```python
from build123d import *

# Parameters (mm, degrees)
PAD_DEPTH       = 74.5
PAD001_DEPTH    = 1
POCKET_DEPTH    = 28.9
POCKET001_DEPTH = 5.001
SKETCH004_R     = 5
POCKET002_DEPTH = 3
SKETCH005_R     = 2
HOLE_DEPTH      = 25
POCKET003_DEPTH = 117.501


with BuildPart() as part:
    # Sketch → Pad (new body)
    with BuildSketch(Plane.XY):
        with BuildLine():
            Line((1, -1), (1, -5))
            Line((1, -5), (114.5, -5))
            Line((114.5, -1), (114.5, -5))
            ThreePointArc((114.5, -1), (115.914212, -0.414215), (116.5, 0.999995))
            Line((116.5, 0.999995), (116.5, 26.9))
            ThreePointArc((116.5, 26.9), (115.914214, 28.314214), (114.5, 28.9))
            Line((1, 28.9), (114.5, 28.9))
            ThreePointArc((1, 28.9), (-0.414214, 28.314214), (-1, 26.9))
            Line((-1, 1), (-1, 26.9))
            ThreePointArc((-1, 1), (-0.414214, -0.414214), (1, -1))
        make_face()
        with BuildLine():
            Line((1, 0), (114.5, 0))
            ThreePointArc((114.5, 0), (115.207107, 0.292893), (115.5, 1))
            Line((115.5, 1), (115.5, 26.9))
            ThreePointArc((115.5, 26.9), (115.207107, 27.607107), (114.5, 27.9))
            Line((114.5, 27.9), (1, 27.9))
            ThreePointArc((1, 27.9), (0.292893, 27.607107), (0, 26.9))
            Line((0, 26.9), (0, 1))
            ThreePointArc((0, 1), (0.292893, 0.292893), (1, 0))
        make_face(mode=Mode.SUBTRACT)
    extrude(amount=PAD_DEPTH)

    # Sketch001 → Pad001 (join)
    with BuildSketch(Plane.XY):
        with BuildLine():
            Line((-1, 1), (-1, 26.9))
            ThreePointArc((1, 28.9), (-0.414214, 28.314214), (-1, 26.9))
            Line((1, 28.9), (114.5, 28.9))
            ThreePointArc((116.5, 26.9), (115.914214, 28.314214), (114.5, 28.9))
            Line((116.5, 26.9), (116.5, 0.999995))
            ThreePointArc((114.5, -1), (115.914212, -0.414215), (116.5, 0.999995))
            Line((114.5, -1), (114.5, -5))
            Line((114.5, -5), (1, -5))
            Line((1, -5), (1, -1))
            ThreePointArc((-1, 1), (-0.414214, -0.414214), (1, -1))
        make_face()
        Polygon((9, 26.9), (9, 1), (106.5, 0.999995), (106.5, 26.9), align=None, mode=Mode.SUBTRACT)
    extrude(amount=PAD001_DEPTH)

    # Sketch002 (on Face22 of Pad001) → Pocket (cut)
    with BuildSketch(Plane(origin=(0, 28.9, 0), x_dir=(-1, 0, 0), z_dir=(0, 1, 0))):
        Polygon((-104.5, 21), (-104.5, 61), (-124.5, 61), (-124.5, 74.5), (9, 74.5), (9, 61), (-11, 61), (-11, 21), align=None)
    extrude(amount=-POCKET_DEPTH, mode=Mode.SUBTRACT)

    # Sketch003 (on Face30 of Pocket) → Pocket001 (cut, through all)
    with BuildSketch(Plane(origin=(0, 0, 0), x_dir=(-1, 0, 0), z_dir=(0, 1, 0))):
        with BuildLine():
            ThreePointArc((-101, 74.5), (-110.545942, 70.545942), (-114.5, 61))
            Line((-114.5, 61), (-124.5, 61))
            Line((-124.5, 61), (-124.5, 74.5))
            Line((-124.5, 74.5), (-101, 74.5))
        make_face()
        with BuildLine():
            ThreePointArc((-1, 61), (-4.954058, 70.545942), (-14.5, 74.5))
            Line((-14.5, 74.5), (9, 74.5))
            Line((9, 74.5), (9, 61))
            Line((9, 61), (-1, 61))
        make_face()
    extrude(amount=-POCKET001_DEPTH, mode=Mode.SUBTRACT)

    # Sketch004 (on Face42 of Pocket001) → Pocket002 (cut)
    with BuildSketch(Plane(origin=(0, 0, 0), x_dir=(-1, 0, 0), z_dir=(0, 1, 0))):
        with Locations((-84.5, 41)):
            Circle(SKETCH004_R)
        with Locations((-31, 41)):
            Circle(SKETCH004_R)
    extrude(amount=-POCKET002_DEPTH, mode=Mode.SUBTRACT)

    # Sketch005 (on Face42 of Pocket001) → Hole (cut)
    with BuildSketch(Plane(origin=(0, 0, 0), x_dir=(-1, 0, 0), z_dir=(0, 1, 0))):
        with Locations((-84.5, 41)):
            Circle(SKETCH005_R)
        with Locations((-31, 41)):
            Circle(SKETCH005_R)
    extrude(amount=-HOLE_DEPTH, mode=Mode.SUBTRACT)

    # Sketch006 (on Face21 of Hole) → Pocket003 (cut, through all)
    with BuildSketch(Plane.YZ.offset(116.5)):
        with BuildLine():
            ThreePointArc((9, 11), (10, 10), (11, 11))
            Line((11, 11), (11, 29))
            ThreePointArc((11, 29), (10, 30), (9, 29))
            Line((9, 11), (9, 29))
        make_face()
        with BuildLine():
            ThreePointArc((9, 38), (10, 37), (11, 38))
            Line((11, 38), (11, 56))
            ThreePointArc((11, 56), (10, 57), (9, 56))
            Line((9, 38), (9, 56))
        make_face()
        with BuildLine():
            ThreePointArc((18.6, 11), (19.6, 10), (20.6, 11))
            Line((20.6, 11), (20.6, 29))
            ThreePointArc((20.6, 29), (19.6, 30), (18.6, 29))
            Line((18.6, 11), (18.6, 29))
        make_face()
        with BuildLine():
            ThreePointArc((18.6, 38), (19.6, 37), (20.6, 38))
            Line((20.6, 38), (20.6, 56))
            ThreePointArc((20.6, 56), (19.6, 57), (18.6, 56))
            Line((18.6, 38), (18.6, 56))
        make_face()
    extrude(amount=-POCKET003_DEPTH, mode=Mode.SUBTRACT)


solid = part.part
```
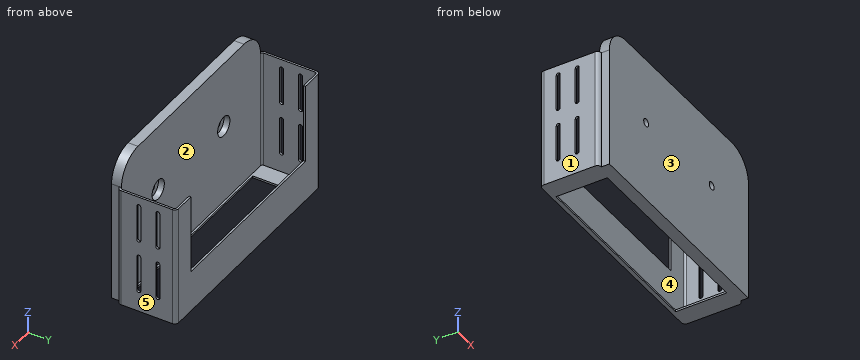
Part model, mm, in its own coordinate system. Face numbers are marked on the shaded views. A direction names the side the tool comes from. Round coordinates to 2 decimals unless told otherwise and drop trailing zeros. Write each loop counter-clockwise with the first axis right and the second up, starting at its lowest first coordinate (ties: lowest second). Pieces come first, ordered by that corner, then holes. Notation, with made-up numbers: M 85.5,10.25 L 135.5,10.25 A19 cw 135.5,20.25 Z; hole C -34,-38 d4. An arc over 180 degrees is marked long. Answer as CSV lines item,"result". Start each with the question number.
1) Mould opens along Y. For the marked faces 1, 2 and 3 say: +Y half, -Y half, draft (parallel to the pull), parting line (faces both ways), or undercut.
2) Which spindle directions (+Z, -Z, +X, -X, +Y, -Y) get a long thin tool onto all of the face, cutting with end or side? Do the marked faces 4 and 5. Say none if no direction does.
3) Band-saw the part on B-B (z = 8). List the corners of the cut face in (x, y), then the cut area to 3 significant figures.
4) Drill centre lines: L1, parallel to X at y = 17, z = 54; L2, parallel to Y at x = 111, z = 25; L3, parallel to Z at x = 31, y = -2. Where is each one in solid material? Low to high.
5) Band-saw the part on A-A (x = 49). List the corners of the cut face in (y, z).
6) Band-saw the part on C-C (z = 41). Count the separate pieces of the cut face and the enclosed holes in it, then the cut area to 3 significant figures.
7) Drop flat-ended pins along their axis: pin 1 (5 mm diameter, centred on x = 87, z = 40, fed in from +Y); pin 2 (13 mm diameter, centred on x = 110.5, y = 21.5, fed in from +Z); pin 3 (0.8 mm diameter, centred on x = 116, z = 23.5, fed in from -Y). Give the stop position or say it passes through.
Worked out:
1,face 1,"draft"
1,face 2,"undercut"
1,face 3,"-Y half"
2,face 4,"+Z"
2,face 5,"+Z, -Z, +X, +Y, -Y"
3,outline,"M -1,1 A2 ccw 1,-1 L 1,-5 L 114.5,-5 L 114.5,-1 A2 ccw 116.5,1 L 116.5,26.9 A2 ccw 114.5,28.9 L 1,28.9 A2 ccw -1,26.9 Z; hole M 0,1 A1 ccw 1,0 L 114.5,0 A1 ccw 115.5,1 L 115.5,26.9 A1 ccw 114.5,27.9 L 1,27.9 A1 ccw 0,26.9 Z"
3,area,"742 mm²"
4,L1,"-1 to 0, 115.5 to 116.5"
4,L2,"-5 to 0, 27.9 to 28.9"
4,L3,"0 to 36, 46 to 74.5"
5,outline,"M -5,0 L 1,0 L 1,1 L 0,1 L 0,74.5 L -5,74.5 Z; M 26.9,0 L 28.9,0 L 28.9,21 L 27.9,21 L 27.9,1 L 26.9,1 Z"
6,separate pieces,"7"
6,enclosed holes,"0"
6,area,"565 mm²"
7,pin 1,"y = 0"
7,pin 2,"z = 61"
7,pin 3,"y = -0.67"
